Check sheet for the modelled part. Datum: model origin and axes. Units: mm. A direction names the side the tool comes from. Coordinates: 2 decimals unless noted, no trailing zeros. Write each loop counter-clockwise with the first axis right and the second up, starting at its lowest first coordinate (ties: lowest second). Pieces come first, ordered by that corner, then holes. Notation, with made-up numbers: M 59,24 L 89,24 A18 ccw 89,30 Z; hole C 45.5,-16 d11. An arc over 180 degrees is marked long. Answer as CSV lines item,"result". Start each with the question number.
1) Section check A-A (z = 23.65). Record the cut outline in (x, y).
2) Go/stop test with flat-tipped pins: pin 1 Ø12 at (y, z) = (18, 1) entering from +X; pin 2 Ø1.5 at (y, z) = (21.5, 1.5) entering from -X; pin 3 Ø4 at (x, z) = (-49.05, 23.65) entering from +Y; pin 4 Ø2 at (x, z) = (49.05, -23.65) entering from +Y. Record where each tip stops, or that it passes through.
3) Draft check along Z on faces 1 (the cylindrical face through (-48.38, 0.811, 22.033)), 2 (the flat face through (-1, 14, 28.5)), 3 (the flat face through (45, 15, 0)). Enter one of: +Z half, -Z half, draft (parallel to the pull), parting line (faces both ways), or undercut.
4) Access from +Z, -Z, +X, -X, +Y, -Y to the whole of each face (thin tool, end or side, straight path). Record for faces 4 (the cylindrical face through (-48.524, 0.811, -21.981)), 5 (the flat face through (49, 1.6, 0)), 6 (the flat face through (-45, 15, 0)).
5) Material ranges on L1, parallel to X at y = 1.1, z = -23.65; L2, parallel to X at y = 24.5, z = 7.5; L3, parallel to Y at x = -48, z = 14.5, recorded low to high. Write a range as [from, to].
6) Section check B-B (x = 49.05). Record the cut outline in (y, z).
7) Section check D-D (y = 24.5). Record the cut outline in (x, z).
8) Section check C-C (z = -16.5). Record the cut outline in (x, y).
from build123d import *

# Parameters (mm, degrees)
SKETCH_1_W          = 106
SKETCH_1_H          = 57
EXTRUDE_1_DEPTH     = 1.6
SKETCH_2_R          = 1.75
CUT_EXTRUDE_1_DEPTH = 1.6
SKETCH_3_W          = 90
SKETCH_3_H          = 57
EXTRUDE_2_DEPTH     = 26.4


with BuildPart() as part:
    # 草图1 → 凸台-拉伸1 (new body)
    with BuildSketch(Plane(origin=(0, 0, 0), x_dir=(1, 0, 0), z_dir=(0, 1, 0))):
        Rectangle(SKETCH_1_W, SKETCH_1_H)
    extrude(amount=EXTRUDE_1_DEPTH)

    # 草图2 → 切除-拉伸1 (cut)
    with BuildSketch(Plane(origin=(0, 1.6, 0), x_dir=(1, 0, 0), z_dir=(0, 1, 0))):
        with Locations(Location((-49.05, 23.65, 0), (0, 0, 270))):
            Circle(SKETCH_2_R)
        with Locations(Location((-49.05, -23.65, 0), (0, 0, 90))):
            Circle(SKETCH_2_R)
        with Locations(Location((49.05, -23.65, 0), (0, 0, 270))):
            Circle(SKETCH_2_R)
        with Locations(Location((49.05, 23.65, 0), (0, 0, 90))):
            Circle(SKETCH_2_R)
    extrude(amount=-CUT_EXTRUDE_1_DEPTH, mode=Mode.SUBTRACT)

    # 草图3 → 凸台-拉伸2 (add)
    with BuildSketch(Plane(origin=(0, 1.6, 0), x_dir=(1, 0, 0), z_dir=(0, 1, 0))):
        Rectangle(SKETCH_3_W, SKETCH_3_H)
    extrude(amount=EXTRUDE_2_DEPTH)


solid = part.part
Results found:
1,outline,"M -53,0 L -50.8,0 L -50.8,1.6 L -53,1.6 Z; M -47.3,0 L 47.3,0 L 47.3,1.6 L 45,1.6 L 45,28 L -45,28 L -45,1.6 L -47.3,1.6 Z; M 50.8,0 L 53,0 L 53,1.6 L 50.8,1.6 Z"
2,pin 1,"stops at x = 45"
2,pin 2,"stops at x = -45"
2,pin 3,"stops at y = 1.6"
2,pin 4,"passes through"
3,face 1,"undercut"
3,face 2,"+Z half"
3,face 3,"draft"
4,face 4,"+Y, -Y"
4,face 5,"+Z, -Z, +X, +Y"
4,face 6,"+Z, -Z, -X, +Y"
5,L1,"x = [-53, -50.8], [-47.3, 47.3], [50.8, 53]"
5,L2,"x = [-45, 45]"
5,L3,"y = [0, 1.6]"
6,outline,"M 0,-28.5 L 1.6,-28.5 L 1.6,-25.4 L 0,-25.4 Z; M 0,-21.9 L 1.6,-21.9 L 1.6,21.9 L 0,21.9 Z; M 0,25.4 L 1.6,25.4 L 1.6,28.5 L 0,28.5 Z"
7,outline,"M -45,-28.5 L 45,-28.5 L 45,28.5 L -45,28.5 Z"
8,outline,"M -53,0 L 53,0 L 53,1.6 L 45,1.6 L 45,28 L -45,28 L -45,1.6 L -53,1.6 Z"
